Can you work these out from the model? Positions are in its coordinate system, mm. Give positions to 0.01 mm unless a question says otherwise; leave off trailing zeros. Order: outer loops, then holes, each group sorted by start corner. A loop starts at its lowest first (then second) coordinate and runs counter-clockwise, first axis right, second up. Notation, with made-up numbers: (84.25, -15.5) - (103.25, -15.5) arc R29 ccw to (103.25, 15.5) - close; hole circle Ø1 at (-16, -39.75). An arc over 180 degrees is marked (long way). Return JSON: item names as keys, results as strings.
```python
from build123d import *

# Parameters (mm, degrees)
SKETCH1_W           = 4.5
SKETCH1_H           = 3.9
BOSS_EXTRUDE1_DEPTH = 1.7
SKETCH2_R           = 1.2
BOSS_EXTRUDE2_DEPTH = 1.2
FILLET1_R           = 1.2
SKETCH3_W           = 0.45
SKETCH3_H           = 0.4
BOSS_EXTRUDE3_DEPTH = 12.8


with BuildPart() as part:
    # Sketch1 → Boss-Extrude1 (new body)
    with BuildSketch(Plane.XY):
        Rectangle(SKETCH1_W, SKETCH1_H)
    extrude(amount=-BOSS_EXTRUDE1_DEPTH)

    # Sketch2 → Boss-Extrude2 (add)
    with BuildSketch(Plane.XY):
        with Locations(Location((0, 0.45, 0), (0, 0, 180))):
            Circle(SKETCH2_R)
    extrude(amount=BOSS_EXTRUDE2_DEPTH)

    # Fillet1
    fillet1_edges = [part.edges().sort_by_distance(p)[0] for p in [
        (1.2, 0.45, 1.2),
    ]]
    fillet(fillet1_edges, radius=FILLET1_R - 0.0001)  # a hair under: the kernel refuses the full size

    # Sketch3 → Boss-Extrude3 (add)
    with BuildSketch(Plane.XZ.offset(1.95)):
        with Locations((1.29, -0.7)):
            Rectangle(SKETCH3_W, SKETCH3_H)
    boss_extrude3 = extrude(amount=BOSS_EXTRUDE3_DEPTH)

    # Mirror1: Boss-Extrude3 across plane
    add(boss_extrude3.mirror(Plane(origin=(0, 0, 0), x_dir=(0, 0, 1), z_dir=(1, 0, 0))))


solid = part.part
```
1. Suppose I cut it at B-B (x = -1.9). List the corners of the cut face in (y, z) for me, plus the area to 3 significant figures.
Checks:
{"outline": "(-1.95, -1.7) - (1.95, -1.7) - (1.95, 0) - (-1.95, 0) - close", "area": "6.63 mm^2"}
2. Suppose I cut it at A-A (y = -2.5). List the corners of the cut face in (x, z) for me (3 decimals), plus the area to 3 significant figures.
Checks:
{"outline": "(-1.515, -0.9) - (-1.065, -0.9) - (-1.065, -0.5) - (-1.515, -0.5) - close; (1.065, -0.9) - (1.515, -0.9) - (1.515, -0.5) - (1.065, -0.5) - close", "area": "0.360 mm^2"}
3. If I drill on L1, parallel to X at y = -13, z = -0.55 (3 decimals); L2, parallel to Z at x = 1.3, y = -2; L3, parallel to Y at x = -0.4, z = -0.15, over which ranges is the centre line in solid material (lowest first)? Write a range as [from, to].
Checks:
{"L1": "[-1.515, -1.065], [1.065, 1.515]", "L2": "[-0.9, -0.5]", "L3": "[-1.95, 1.95]"}
4. For pin 1 Ø1 at (x, y) = (-1, -6) entering from -Z, with a flat end and sliding along its axis, tell me the tip position at first contact or that it passes through.
Checks:
{"pin 1": "z = -0.9"}
